Autodesk Inventor part; units mm, degrees
ref_plane "YZ Plane" through (0, 0, 0) normal (1, 0, 0) x (0, 1, 0)
ref_plane "XZ Plane" through (0, 0, 0) normal (0, 1, 0) x (-1, 0, 0)
ref_plane "XY Plane" through (0, 0, 0) normal (0, 0, 1) x (1, 0, 0)
sketch "Sketch1" plane through (0, 0, 0) normal (0, 1, 0) x (-1, 0, 0)
  line L0 (0, 0) -> (-20, 0)
  line L1 (-20, 0) -> (-20, -60)
  line L2 (-20, -60) -> (0, -60)
  line L3 (0, -60) -> (0, 0)
  line L4 (0, -60) -> (-15, -60)
  line L5 (0, -60) -> (15, -60) construction
  line L6 (-15, -60) -> (-15, 0)
  dimension "d0" = 20
  dimension "d1" = 60
  dimension "d14" = 15
  dimension "d15" = 180
extrude "Extrusion1" add sketch "Sketch1" along normal blind 5
sketch "Sketch2" plane through (0, 5, 0) normal (0, 1, 0) x (1, 0, 0)
  line L0 (10, 0) -> (19, 0) construction
  line L1 (0, 0) -> (20, 0)
  line L2 (0, 0) -> (15, 0) construction
  line L3 (7.5, 0) -> (16.5, 0) construction
  line L4 (0, 60) -> (0, 0) construction
  line L5 (7.5, 9) -> (0, 9) construction
  circle A0 centre (7.5, 51) radius 0.425 construction
  line L6 (7.5, 51) -> (1.0192, 51) construction
  line L7 (7.5, 51) -> (7.5, 47.5) construction
  line L8 (7.5, 51) -> (11.5, 51) construction
  ellipse E0 centre (7.5, 51) end of major axis (11.5, 51) minor radius 3.5
  line L9 (20, 0) -> (20, 60) construction
  line L10 (20, 30) -> (0, 30) construction
  ellipse E1 centre (7.5, 9) end of major axis (11.5, 9) minor radius 3.5
  dimension "d30" = 0.85
  dimension "d32" = 3.5
  dimension "d33" = 4
sketch "Sketch3" plane through (0, 5, 0) normal (0, 1, 0) x (1, 0, 0)
  line L0 (0, 60) -> (0, 0)
  line L1 (20, 0) -> (20, 60)
  line L2 (0, 15.7197) -> (20, 15.7197)
  line L3 (20, 15.7197) -> (20, 44.2851)
  line L4 (20, 44.2851) -> (0, 44.2851)
  line L5 (0, 44.2851) -> (0, 15.7197)
extrude "Extrusion3" add sketch "Sketch3" along normal blind 15
sketch "Sketch4" plane through (20, 0, 0) normal (1, 0, 0) x (0, 0, -1)
  line L0 (15.7197, 5) -> (15.7197, 20)
  line L1 (44.2851, 5) -> (60, 5)
  circle A0 centre (30.0024, 12.5) radius 3.75
  point P0 (0, 0)
  dimension "d11" = 7.5
extrude "Extrusion4" cut sketch "Sketch4" against normal blind 65.5
extrude "Extrusion5" add sketch "Sketch1" along normal blind 5 contours L3 L2 L6 L0
extrude "Extrusion6" cut sketch "Sketch1" along normal blind 22.5 contours L6 L2 L1 L0
extrude "Extrusion9" cut sketch "Sketch2" against normal blind 10
properties part number "SuperiorBancada"
Part model, mm, in its own coordinate system. A direction names the side the tool comes from. Round coordinates to 2 decimals unless told otherwise and drop trailing zeros. Loops run counter-clockwise (first coordinate to the right, second up) from the corner with the lowest first, then second, coordinate; pieces in that order, holes last. Notation, with made-up numbers: (1, -37) -> (25, -37) arc R7 ccw to (25, -30) -> close; hole circle Ø8 at (20.5, 51.25). An arc over 180 degrees is marked (long way). Use one line per item in the form item = value. Start each with the question number.
Item 1: Band-saw the part on B-B (x = 13.75). List the corners of the cut face in (y, z), plus the area to 3 significant figures.
Item 2: Band-saw the part on C-C (z = -31.5). List the corners of the cut face in (x, y).
Item 3: Two-plate mould, pull along Z, no slides. Class faces 1 (the flat face through (8, 12, -44.285)), 2 (the cylindrical face through (7.605, 12.665, -26.256)), 3 (the flat face through (7, 2, 0)): released by +Z, released by -Z, zero draft, split by the parting line, or undercut.
Item 4: Band-saw the part on A-A (y = 12.5). List the corners of the cut face in (x, z).
Item 5: Tool access for faces 4 (the flat face through (8, 5, -4)), 5 (the flat face through (8, 5, -56)), 6 (the flat face through (8, 0, -30)): list every direction of +Z, -Z, +X, -X, +Y, -Y with a clear straight run to the whole face (end or side of a thin tool).
Item 6: Drop flat-ended pins along their axis: pin 1 Ø4 at (x, y) = (11.5, 8.5) entering from +Z; pin 2 Ø1 at (x, z) = (8, -6) entering from +Y; pin 3 Ø4.5 at (x, y) = (6, 13.5) entering from -Z. Give the stop position or say it passes through.
Item 7: Band-saw the part on D-D (x = 6.25). Give the number of separate pieces and of enclosed holes in the cut face, plus the area to 3 significant figures.
Item 8: Drill centre lines: line 1 along Z through (x, y) = (1.75, 8); line 2 along Z through (x, y) = (5.25, 2.5); line 3 along Y through (x, z) = (4.5, -56.5). Where is each one in solid material? Low to high.
Data:
q1.outline = (0, -60) -> (5, -60) -> (5, -44.29) -> (20, -44.29) -> (20, -15.72) -> (5, -15.72) -> (5, 0) -> (0, 0) -> close; hole circle Ø7.5 at (12.5, -30)
q1.area = 684 mm^2
q2.outline = (0, 0) -> (15, 0) -> (15, 9.06) -> (0, 9.06) -> close; (0, 15.94) -> (15, 15.94) -> (15, 20) -> (0, 20) -> close
q3.face_1 = released by -Z
q3.face_2 = undercut
q3.face_3 = released by +Z
q4.outline = (0, -44.29) -> (15, -44.29) -> (15, -33.75) -> (0, -33.75) -> close; (0, -26.25) -> (15, -26.25) -> (15, -15.72) -> (0, -15.72) -> close
q5.face_4 = +Z, +X, -X, +Y
q5.face_5 = -Z, +X, -X, +Y
q5.face_6 = +Z, -Z, +X, -X, -Y
q6.pin_1 = -15.72
q6.pin_2 = 5
q6.pin_3 = -44.29
q7.separate_pieces = 3
q7.enclosed_holes = 1
q7.area = 618 mm^2
q8.line_1 = -44.29 to -15.72
q8.line_2 = -60 to -53.89, -48.11 to -11.89, -6.11 to 0
q8.line_3 = 0 to 5
